```python
from build123d import *

# Parameters (mm, degrees)
F2_SIZE = 1


with BuildPart() as f1:
    # F0 (on Right) → F1 (revolve)
    with BuildSketch(Plane.YZ):
        Polygon((0, 6), (4, 6), (4, 2.5), (7, 2.5), (7, 11), (2, 11), (2, 12.5), (0, 12.5), align=None)
    revolve(axis=Axis((0, 5.735075, 0), (0, -1, 0)))

    # F2
    f2_edges = [f1.edges().sort_by_distance(p)[0] for p in [
        (0, 7, -11),
    ]]
    chamfer(f2_edges, length=F2_SIZE)


solid = f1.part
```
Can you work these out from the model? Positions are in its coordinate system, mm. A direction names the side the tool comes from. Coordinates: 2 decimals unless noted, no trailing zeros. Loops run counter-clockwise (first coordinate to the right, second up) from the corner with the lowest first, then second, coordinate; pieces in that order, holes last. Notation, with made-up numbers: (-13, -25) -> (-3, -25) arc R6 ccw to (-3, -20) -> close; hole circle Ø11 at (81.5, 1). An arc over 180 degrees is marked (long way). Put each result on its own line as item: value. Start each with the question number.
Q1. I want a section at D-D (y = 1). Write out the boundary of the cut face in (x, z), plus the area to 3 significant figures.
Q2. For faces 1 (the face through (5.4, 0, -3)), 2 (the face through (0, 2, -6)), which set-ups out of +Z, -Z, +X, -X, +Y, -Y let a thin tool reach every point of the face, with its end or its side?
Q3. If I drill on line 1 (X direction, y = 1.8, z = 0); line 2 (X direction, y = 5.9, z = 0), over which ranges is the centre line in solid material (lowest first)? Write a range as [from, to].
Q4. I want a section at C-C (y = 5). Write out the boundary of the cut face in (x, z), plus the area to 3 significant figures.
Q5. Thinking about a two-plate mould opening in Z: for faces 3 (the face through (10.74, 3.97, -2.38)), 4 (the face through (2.44, 5.52, -0.54)), 5 (the face through (0, 4, 3)), 6 (the face through (10, 2, -5)), which applies, pulls with the +Z half, pulls with the -Z half, needs draft (parallel to the pull), parting line crosses it, or undercut?
Q6. I want a section at A-A (x = 0). Write out the boundary of the cut face in (y, z), plus the area to 3 significant figures.
Q7. I'm going to push flat-ended pins straight in: P1, Ø7, axis at x = 0, z = 0, coming from the +Y side; P2, Ø3, axis at x = 6, y = 4.5, coming from the -Z side; P3, Ø1, axis at x = 5.5, y = 2, coming from the +Z side. Where does each tip first touch, or does it pass through?
Q8. I want a section at B-B (z = 0). Write out the boundary of the cut face in (x, y).
Taken from the geometry:
1. outline: circle Ø25 at (0, 0); hole circle Ø12 at (0, 0)
1. area: 378 mm2
2. face 1: +Z, -Z, +X, -X, -Y
2. face 2: -Y
3. line 1: x = [-12.5, -6], [6, 12.5]
3. line 2: x = [-11, -2.5], [2.5, 11]
4. outline: circle Ø22 at (0, 0); hole circle Ø5 at (0, 0)
4. area: 360 mm2
5. face 3: parting line crosses it
5. face 4: undercut
5. face 5: undercut
5. face 6: needs draft
6. outline: (0, -12.5) -> (2, -12.5) -> (2, -11) -> (6, -11) -> (7, -10) -> (7, -2.5) -> (4, -2.5) -> (4, -6) -> (0, -6) -> close; (0, 6) -> (4, 6) -> (4, 2.5) -> (7, 2.5) -> (7, 10) -> (6, 11) -> (2, 11) -> (2, 12.5) -> (0, 12.5) -> close
6. area: 96.0 mm2
7. P1: stops at y = 7
7. P2: stops at z = -10.04
7. P3: stops at z = 11.46
8. outline: (-12.5, 0) -> (-6, 0) -> (-6, 4) -> (-2.5, 4) -> (-2.5, 7) -> (-10, 7) -> (-11, 6) -> (-11, 2) -> (-12.5, 2) -> close; (2.5, 4) -> (6, 4) -> (6, 0) -> (12.5, 0) -> (12.5, 2) -> (11, 2) -> (11, 6) -> (10, 7) -> (2.5, 7) -> close
